```python
from build123d import *

# Parameters (mm, degrees)
SKETCH1_R           = 25
SKETCH1_R_2         = 1.6
BOSS_EXTRUDE1_DEPTH = 4.7625


with BuildPart() as part:
    # Sketch1 → Boss-Extrude1 (new body)
    with BuildSketch(Plane(origin=(0, 0, 0), x_dir=(1, 0, 0), z_dir=(0, 1, 0))):
        Circle(SKETCH1_R)
        with Locations((20, 0)):
            Circle(SKETCH1_R_2, mode=Mode.SUBTRACT)
        with Locations((12, 0)):
            Circle(SKETCH1_R_2, mode=Mode.SUBTRACT)
        with Locations((17.320508076, -10)):
            Circle(SKETCH1_R_2, mode=Mode.SUBTRACT)
        with Locations((10.392304845, -6)):
            Circle(SKETCH1_R_2, mode=Mode.SUBTRACT)
        with Locations((10, -17.320508076)):
            Circle(SKETCH1_R_2, mode=Mode.SUBTRACT)
        with Locations((6, -10.392304845)):
            Circle(SKETCH1_R_2, mode=Mode.SUBTRACT)
        with Locations((0, -20)):
            Circle(SKETCH1_R_2, mode=Mode.SUBTRACT)
        with Locations((0, -12)):
            Circle(SKETCH1_R_2, mode=Mode.SUBTRACT)
        with Locations((-10, -17.320508076)):
            Circle(SKETCH1_R_2, mode=Mode.SUBTRACT)
        with Locations((-6, -10.392304845)):
            Circle(SKETCH1_R_2, mode=Mode.SUBTRACT)
        with Locations((-17.320508076, -10)):
            Circle(SKETCH1_R_2, mode=Mode.SUBTRACT)
        with Locations((-10.392304845, -6)):
            Circle(SKETCH1_R_2, mode=Mode.SUBTRACT)
        with Locations((-20, 0)):
            Circle(SKETCH1_R_2, mode=Mode.SUBTRACT)
        with Locations((-12, 0)):
            Circle(SKETCH1_R_2, mode=Mode.SUBTRACT)
        with Locations((-17.320508076, 10)):
            Circle(SKETCH1_R_2, mode=Mode.SUBTRACT)
        with Locations((-10.392304845, 6)):
            Circle(SKETCH1_R_2, mode=Mode.SUBTRACT)
        with Locations((-10, 17.320508076)):
            Circle(SKETCH1_R_2, mode=Mode.SUBTRACT)
        with Locations((-6, 10.392304845)):
            Circle(SKETCH1_R_2, mode=Mode.SUBTRACT)
        with Locations((0, 20)):
            Circle(SKETCH1_R_2, mode=Mode.SUBTRACT)
        with Locations((0, 12)):
            Circle(SKETCH1_R_2, mode=Mode.SUBTRACT)
        with Locations((10, 17.320508076)):
            Circle(SKETCH1_R_2, mode=Mode.SUBTRACT)
        with Locations((6, 10.392304845)):
            Circle(SKETCH1_R_2, mode=Mode.SUBTRACT)
        with Locations((17.320508076, 10)):
            Circle(SKETCH1_R_2, mode=Mode.SUBTRACT)
        with Locations((10.392304845, 6)):
            Circle(SKETCH1_R_2, mode=Mode.SUBTRACT)
    extrude(amount=BOSS_EXTRUDE1_DEPTH)


solid = part.part
```
Geometry: final body of the model. Coordinates: model frame, mm. Coordinates: 2 decimals unless noted, no trailing zeros. Order: outer loops, then holes, each group sorted by start corner. A loop starts at its lowest first (then second) coordinate and runs counter-clockwise, first axis right, second up.
Item 1: Contact query for flat-ended pins moving along their axis: P1, Ø5, axis at x = 10.39, z = -6, coming from the +Y side; P2, Ø1, axis at y = 3.5, z = 1, coming from the -X side (3 decimals); P3, Ø1, axis at y = 2, z = -13, coming from the -X side; P4, Ø1.5, axis at x = 7, y = 2, coming from the +Z side. Output: stop coordinate, or through.
Answer:
P1: stops at y = 4.76
P2: stops at x = -24.995
P3: stops at x = -21.65
P4: stops at z = 24.21
Item 2: Draft query along Z for faces 1 (the face through (0, 4.762, 0)), 2 (the face through (-0.208, 2.348, -13.586)). Return one class per face: released by +Z, released by -Z, zero draft, split by the parting line, or undercut.
Answer:
face 1: zero draft
face 2: undercut
Item 3: Section query D-D (z = -6). Output: boundary loops of the cut face in (x, y).
Answer:
outline: (-24.27, 0) - (-11.99, 0) - (-11.99, 4.76) - (-24.27, 4.76) - close; (-8.79, 0) - (8.79, 0) - (8.79, 4.76) - (-8.79, 4.76) - close; (11.99, 0) - (24.27, 0) - (24.27, 4.76) - (11.99, 4.76) - close
Item 4: Section query B-B (x = -13). Output: boundary loops of the cut face in (y, z), then the cut area to 3 significant figures.
Answer:
outline: (0, -21.35) - (4.76, -21.35) - (4.76, -1.25) - (0, -1.25) - close; (0, 1.25) - (4.76, 1.25) - (4.76, 21.35) - (0, 21.35) - close
area: 192 mm2
Item 5: Material intervals for line 1 along X through (y, z) = (3.45, 0); line 2 along Z through (x, y) = (-5, 4.1), sorted ascending.
Answer:
line 1: x = -25 to -21.6, -18.4 to -13.6, -10.4 to 10.4, 13.6 to 18.4, 21.6 to 25
line 2: z = -24.49 to -11.64, -9.14 to 9.14, 11.64 to 24.49
Item 6: Section query C-C (y = 3.7). State how many separate pieces and enclosed holes the cut face has, then the cut area to 3 significant figures.
Answer:
separate pieces: 1
enclosed holes: 24
area: 1,770 mm2
Item 7: Section query A-A (z = 0). Output: boundary loops of the cut face in (x, y).
Answer:
outline: (-25, 0) - (-21.6, 0) - (-21.6, 4.76) - (-25, 4.76) - close; (-18.4, 0) - (-13.6, 0) - (-13.6, 4.76) - (-18.4, 4.76) - close; (-10.4, 0) - (10.4, 0) - (10.4, 4.76) - (-10.4, 4.76) - close; (13.6, 0) - (18.4, 0) - (18.4, 4.76) - (13.6, 4.76) - close; (21.6, 0) - (25, 0) - (25, 4.76) - (21.6, 4.76) - close
